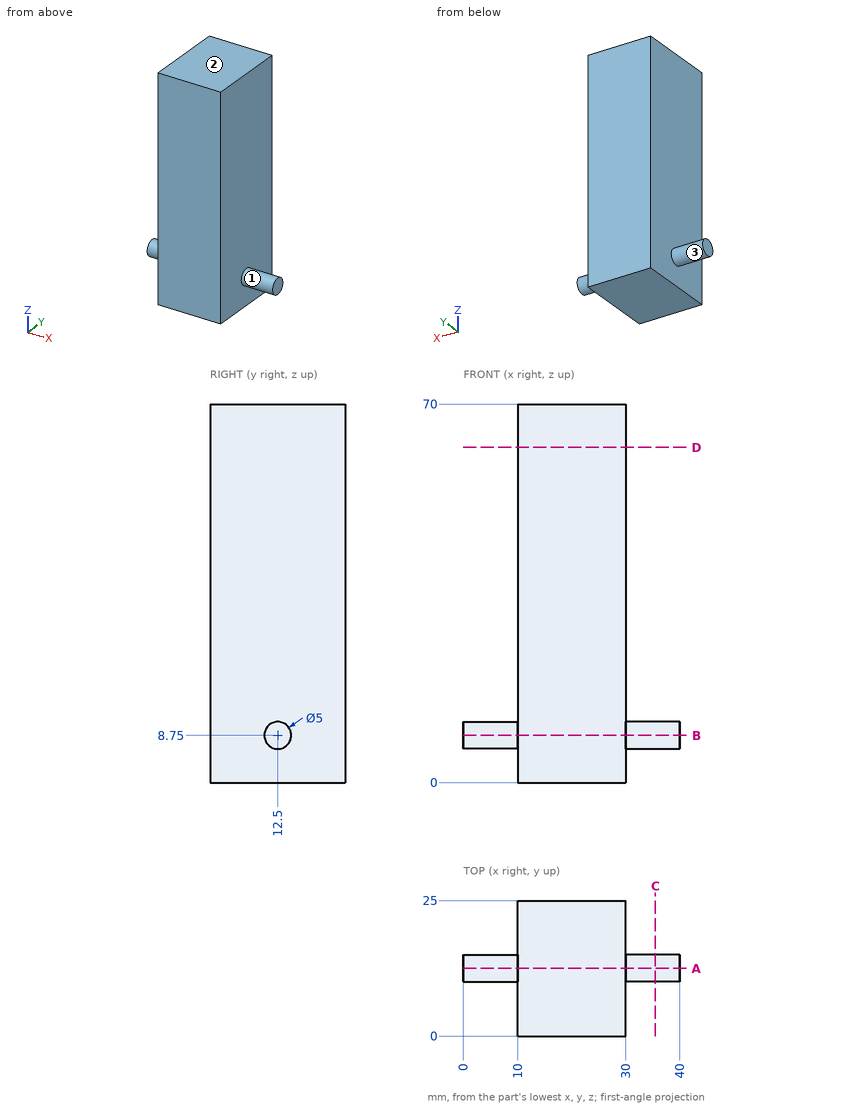
The drawing under review shows one solid part. Ordinate dimensions are in mm from its lowest x, y, z. A direction names the side the tool comes from. Coordinates: 2 decimals unless noted, no trailing zeros. Order: outer loops, then holes, each group sorted by start corner. A loop starts at its lowest first (then second) coordinate and runs counter-clockwise, first axis right, second up. Notation, with made-up numbers: (67.5, -35) -> (126.5, -35) arc R15 ccw to (126.5, -21) -> close; hole circle Ø5 at (58.5, 18.25). An arc over 180 degrees is marked (long way). Return JSON: item names as keys, results as strings.
1. For line 1 (X direction, y = 12.75, z = 21); line 2 (Z direction, x = 4, y = 11.25), list the stretches that pass through material, from the lowest coordinate up. Write a range as from..to.
Answer block:
{"line 1": "10..30", "line 2": "6.58..10.92"}
2. We need section C-C on x = 35.5. Write out the cut boundary in (y, z).
Answer block:
{"outline": "circle Ø5 at (12.5, 8.75)"}
3. We need section B-B on z = 8.75. Write out the cut boundary in (x, y).
Answer block:
{"outline": "(0, 10) -> (10, 10) -> (10, 0) -> (30, 0) -> (30, 10) -> (40, 10) -> (40, 15) -> (30, 15) -> (30, 25) -> (10, 25) -> (10, 15) -> (0, 15) -> close"}
4. We need section D-D on z = 62. Write out the cut boundary in (x, y), and give its area (3 significant figures).
Answer block:
{"outline": "(10, 0) -> (30, 0) -> (30, 25) -> (10, 25) -> close", "area": "500 mm²"}
5. Machinability: for the marked faces 1, 2 and 3, which of the approach directions +Z, -Z, +X, -X, +Y, -Y give a long, thin tool a straight path to every point of the face, cutting with its end or side? Answer none if there is none.
Answer block:
{"face 1": "+X", "face 2": "+Z, +X, -X, +Y, -Y", "face 3": "-X"}
6. For pin 1 Ø10 at (y, z) = (14.5, 35) entering from -X; pin 2 Ø5 at (y, z) = (10, 30) entering from +X, all flat-tipped, find the tip position at first contact; note any pin that passes through.
Answer block:
{"pin 1": "x = 10", "pin 2": "x = 30"}
7. We need section A-A on y = 12.5. Write out the cut boundary in (x, z), and give its area (3 significant figures).
Answer block:
{"outline": "(0, 6.25) -> (10, 6.25) -> (10, 0) -> (30, 0) -> (30, 6.25) -> (40, 6.25) -> (40, 11.25) -> (30, 11.25) -> (30, 70) -> (10, 70) -> (10, 11.25) -> (0, 11.25) -> close", "area": "1,500 mm²"}
